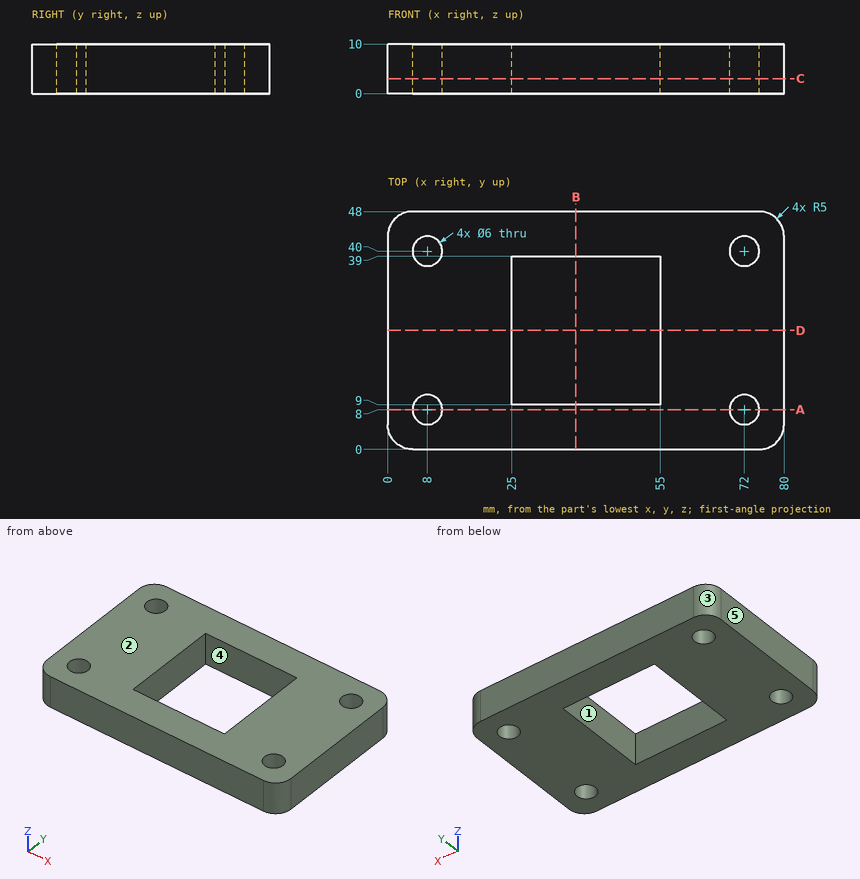
For this review, use the dimensioned drawing (mm, ordinates from the lowest corner) and the shaded views. A direction names the side the tool comes from. Coordinates: 2 decimals unless noted, no trailing zeros. Loops run counter-clockwise (first coordinate to the right, second up) from the corner with the lowest first, then second, coordinate; pieces in that order, holes last. Notation, with made-up numbers: (2, -25.75) -> (59, -25.75) arc R30 ccw to (59, -2.75) -> close; hole circle Ø6 at (56, -19.75). An arc over 180 degrees is marked (long way). Return JSON: item names as keys, results as strings. Group by question number.
(1) For pin 1 Ø5.5 at (x, y) = (8, 8) entering from -Z, flat-tipped, find the tip position at first contact; note if it passes through.
(2) Consider section B-B, the plane x = 38. Give the boundary of the cut face in (y, z), plus the area to 3 significant figures.
(3) Consider section A-A, the plane y = 8. Give the boundary of the cut face in (x, z).
(4) Consider section C-C, the plane z = 3. Give the boundary of the cut face in (x, y), plus the area to 3 significant figures.
(5) To check wall thickness, follow L1, parallel to Y at x = 8, z = 5; L2, parallel to X at y = 40, z = 7.5; L3, parallel to X at y = 19, z = 3.5. State the ranges of each line that lie inside material, in increasing order.
(6) Consider section D-D, the plane y = 24. Give the boundary of the cut face in (x, z).
(7) Mouldability with a two-part tool opening along X and no side actions: class the marked faces 1, 2 and 3 as pulls with the +X half, pulls with the -X half, needs draft (parallel to the pull), parting line crosses it, or undercut.
(8) Tool access review of the marked faces 4 and 5: name each direction out of +Z, -Z, +X, -X, +Y, -Y from which nothing blocks a thin tool from reaching the whole face with its end or side.
Results below:
{
 "1": {"pin 1": "passes through"},
 "2": {"outline": "(0, 0) -> (9, 0) -> (9, 10) -> (0, 10) -> close; (39, 0) -> (48, 0) -> (48, 10) -> (39, 10) -> close", "area": "180 mm2"},
 "3": {"outline": "(0, 0) -> (5, 0) -> (5, 10) -> (0, 10) -> close; (11, 0) -> (69, 0) -> (69, 10) -> (11, 10) -> close; (75, 0) -> (80, 0) -> (80, 10) -> (75, 10) -> close"},
 "4": {"outline": "(0, 5) arc R5 ccw to (5, 0) -> (75, 0) arc R5 ccw to (80, 5) -> (80, 43) arc R5 ccw to (75, 48) -> (5, 48) arc R5 ccw to (0, 43) -> close; hole circle Ø6 at (8, 8); hole circle Ø6 at (8, 40); hole (25, 9) -> (55, 9) -> (55, 39) -> (25, 39) -> close; hole circle Ø6 at (72, 8); hole circle Ø6 at (72, 40)", "area": "2,810 mm2"},
 "5": {"L1": "y = 0 to 5, 11 to 37, 43 to 48", "L2": "x = 0 to 5, 11 to 69, 75 to 80", "L3": "x = 0 to 25, 55 to 80"},
 "6": {"outline": "(0, 0) -> (25, 0) -> (25, 10) -> (0, 10) -> close; (55, 0) -> (80, 0) -> (80, 10) -> (55, 10) -> close"},
 "7": {"face 1": "undercut", "face 2": "needs draft", "face 3": "pulls with the -X half"},
 "8": {"face 4": "+Z, -Z", "face 5": "+Z, -Z, -X, +Y, -Y"}
}
